from build123d import *

# Parameters (mm, degrees)
F0_W            = 19.812
F0_H            = 19.812
F1_DEPTH        = 31.9532
F2_R            = 3.556
F3_DEPTH        = 25.9334
F4_T1_DEPTH     = 0.8065583261
F4_T3_DEPTH     = 0.8065583261
F4_T5_DEPTH     = 0.8065583261
F4_T7_DEPTH     = 0.8065583261
F4_T9_DEPTH     = 0.8065583261
F4_T11_DEPTH    = 0.8065583261
F4_T13_DEPTH    = 0.8065583261
F4_T15_DEPTH    = 0.8065583261
F4_T17_DEPTH    = 35.2192373947
F4_T19_DEPTH    = 23.0780373947
F4_T21_DEPTH    = 23.0780373947
F5_W            = 0.254
F5_H            = 11.8872
F5_H_2          = 0.254
F5_W_2          = 9.779
F5_H_3          = 19.812
F6_DEPTH        = 1.016
F6_COPIES_COUNT = 4
F7_W            = 0.254
F7_H            = 8.763
F7_H_2          = 0.254
F7_W_2          = 8.763
F8_DEPTH        = 1.016


# Not quite as in the source:
# - a fillet or chamfer that OpenCascade refuses, or shapes differently, is made with other operations: its cross-section is extruded or revolved along the edge and cut away or added
# - a pattern or mirror of a feature is missing from the dataset's text; its kind, count and spacing are read off the source's solid


with BuildPart() as f1:
    # F0 (on Top) → F1 (new body)
    with BuildSketch(Plane.XY):
        Rectangle(F0_W, F0_H)
    extrude(amount=F1_DEPTH)

    # F2 (on face) → F3 (cut)
    with BuildSketch(Plane.XY.offset(31.9532)):
        Circle(F2_R)
    extrude(amount=-F3_DEPTH, mode=Mode.SUBTRACT)

    # F4: chamfer of 0.635 on 12 edges, made by hand

    # F4_s2 → F4_t1 (cut)
    with BuildSketch(Plane(origin=(-6.1806666667, 6.1806666667, -6.1806666667), x_dir=(-0.7071067812, -0.7071067812, 0), z_dir=(-0.5773502692, 0.5773502692, -0.5773502692))):
        Polygon((-0.4490128061, 8.3474527951), (0, 7.5697398018), (0.4490128061, 8.3474527951), align=None)
    extrude(amount=F4_T1_DEPTH, mode=Mode.SUBTRACT)

    # F4_s4 → F4_t3 (cut)
    with BuildSketch(Plane(origin=(-16.8317333333, 16.8317333333, 16.8317333333), x_dir=(-0.7071067812, -0.7071067812, 0), z_dir=(-0.5773502692, 0.5773502692, 0.5773502692))):
        Polygon((-0.4490128061, 17.7422257546), (0, 18.5199387479), (0.4490128061, 17.7422257546), align=None)
    extrude(amount=F4_T3_DEPTH, mode=Mode.SUBTRACT)

    # F4_s6 → F4_t5 (cut)
    with BuildSketch(Plane(origin=(-6.1806666667, -6.1806666667, -6.1806666667), x_dir=(0.7071067812, -0.7071067812, 0), z_dir=(-0.5773502692, -0.5773502692, -0.5773502692))):
        Polygon((0.4490128061, 8.3474527951), (0, 7.5697398018), (-0.4490128061, 8.3474527951), align=None)
    extrude(amount=F4_T5_DEPTH, mode=Mode.SUBTRACT)

    # F4_s8 → F4_t7 (cut)
    with BuildSketch(Plane(origin=(-16.8317333333, -16.8317333333, 16.8317333333), x_dir=(0.7071067812, -0.7071067812, 0), z_dir=(-0.5773502692, -0.5773502692, 0.5773502692))):
        Polygon((0.4490128061, 17.7422257546), (0, 18.5199387479), (-0.4490128061, 17.7422257546), align=None)
    extrude(amount=F4_T7_DEPTH, mode=Mode.SUBTRACT)

    # F4_s10 → F4_t9 (cut)
    with BuildSketch(Plane(origin=(6.1806666667, -6.1806666667, -6.1806666667), x_dir=(0.7071067812, 0.7071067812, 0), z_dir=(0.5773502692, -0.5773502692, -0.5773502692))):
        Polygon((0.4490128061, 8.3474527951), (-0.4490128061, 8.3474527951), (0, 7.5697398018), align=None)
    extrude(amount=F4_T9_DEPTH, mode=Mode.SUBTRACT)

    # F4_s12 → F4_t11 (cut)
    with BuildSketch(Plane(origin=(16.8317333333, -16.8317333333, 16.8317333333), x_dir=(0.7071067812, 0.7071067812, 0), z_dir=(0.5773502692, -0.5773502692, 0.5773502692))):
        Polygon((0.4490128061, 17.7422257546), (-0.4490128061, 17.7422257546), (0, 18.5199387479), align=None)
    extrude(amount=F4_T11_DEPTH, mode=Mode.SUBTRACT)

    # F4_s14 → F4_t13 (cut)
    with BuildSketch(Plane(origin=(6.1806666667, 6.1806666667, -6.1806666667), x_dir=(-0.7071067812, 0.7071067812, 0), z_dir=(0.5773502692, 0.5773502692, -0.5773502692))):
        Polygon((-0.4490128061, 8.3474527951), (0.4490128061, 8.3474527951), (0, 7.5697398018), align=None)
    extrude(amount=F4_T13_DEPTH, mode=Mode.SUBTRACT)

    # F4_s16 → F4_t15 (cut)
    with BuildSketch(Plane(origin=(16.8317333333, 16.8317333333, 16.8317333333), x_dir=(-0.7071067812, 0.7071067812, 0), z_dir=(0.5773502692, 0.5773502692, 0.5773502692))):
        Polygon((-0.4490128061, 17.7422257546), (0.4490128061, 17.7422257546), (0, 18.5199387479), align=None)
    extrude(amount=F4_T15_DEPTH, mode=Mode.SUBTRACT)

    # F4_s18 → F4_t17 (cut)
    with BuildSketch(Plane.XY.offset(-1.6330186974)):
        Polygon((-9.271, 9.906), (-9.906, 9.271), (-9.906, 9.906), align=None)
        Polygon((-9.271, -9.906), (-9.906, -9.271), (-9.906, -9.906), align=None)
        Polygon((9.906, -9.271), (9.271, -9.906), (9.906, -9.906), align=None)
        Polygon((9.906, 9.271), (9.271, 9.906), (9.906, 9.906), align=None)
    extrude(amount=F4_T17_DEPTH, mode=Mode.SUBTRACT)

    # F4_s20 → F4_t19 (cut)
    with BuildSketch(Plane.XZ.offset(-11.5390186974)):
        Polygon((9.906, 31.3182), (9.271, 31.9532), (9.906, 31.9532), align=None)
        Polygon((-9.271, 31.9532), (-9.906, 31.3182), (-9.906, 31.9532), align=None)
        Polygon((9.906, 0.635), (9.271, 0), (9.906, 0), align=None)
        Polygon((-9.271, 0), (-9.906, 0.635), (-9.906, 0), align=None)
    extrude(amount=F4_T19_DEPTH, mode=Mode.SUBTRACT)

    # F4_s22 → F4_t21 (cut)
    with BuildSketch(Plane.YZ.offset(-11.5390186974)):
        Polygon((-9.906, 31.3182), (-9.271, 31.9532), (-9.906, 31.9532), align=None)
        Polygon((9.906, 31.3182), (9.271, 31.9532), (9.906, 31.9532), align=None)
        Polygon((9.906, 0.635), (9.271, 0), (9.906, 0), align=None)
        Polygon((-9.906, 0.635), (-9.271, 0), (-9.906, 0), align=None)
    extrude(amount=F4_T21_DEPTH, mode=Mode.SUBTRACT)

    # F5 (on face) → F6 (cut)
    with BuildSketch(Plane.XZ.offset(9.906)):
        with Locations((0, 26.0096)):
            Rectangle(F5_W, F5_H)
        with Locations((0, 19.939)):
            Rectangle(F5_W, F5_H_2)
        with Locations((-5.0165, 19.939)):
            Rectangle(F5_W_2, F5_H_2)
        with Locations((5.0165, 19.939)):
            Rectangle(F5_W_2, F5_H_2)
        with Locations((0, 9.906)):
            Rectangle(F5_W, F5_H_3)
    f6 = extrude(amount=-F6_DEPTH, mode=Mode.SUBTRACT)

    # F6_copies: F6 ×4 about axis
    f6_copies_axis = Axis((0, 0, 0), (0, 0, 1))
    for i in range(1, F6_COPIES_COUNT):
        add(f6.rotate(f6_copies_axis, i * 360 / F6_COPIES_COUNT), mode=Mode.SUBTRACT)

    # F7 (on face) → F8 (cut)
    with BuildSketch(Plane(origin=(0, 0, 0), x_dir=(1, 0, 0), z_dir=(0, 0, -1))):
        with Locations((0, 4.5085)):
            Rectangle(F7_W, F7_H)
        Rectangle(F7_W, F7_H_2)
        with Locations((-4.5085, 0)):
            Rectangle(F7_W_2, F7_H_2)
        with Locations((4.5085, 0)):
            Rectangle(F7_W_2, F7_H_2)
        with Locations((0, -4.5085)):
            Rectangle(F7_W, F7_H)
    extrude(amount=-F8_DEPTH, mode=Mode.SUBTRACT)


solid = f1.part
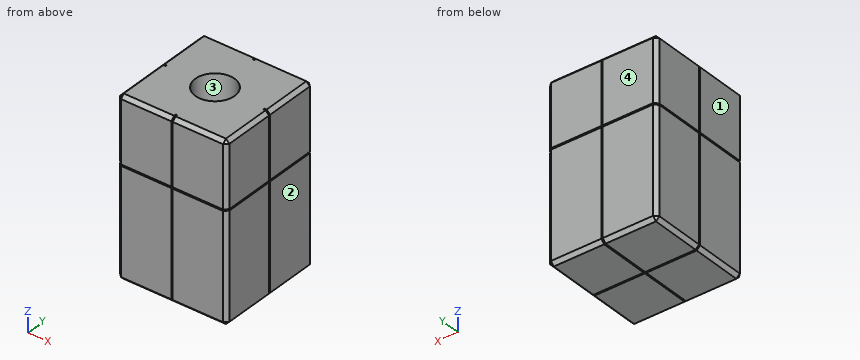
CAD build for the part. Positions are in the model's coordinates, mm. Face numbers are marked on the shaded views. Give positions to 0.01 mm unless a question says otherwise; leave off trailing zeros. Write each loop counter-clockwise with the first axis right and the second up, starting at its lowest first coordinate (ties: lowest second). Pieces come first, ordered by that corner, then holes. Notation, with made-up numbers: (53.25, 53.25) -> (108.25, 53.25) arc R23 ccw to (108.25, 72.25) -> close; hole circle Ø9 at (45, 29.5). An arc over 180 degrees is marked (long way). Return JSON: item names as keys, results as strings.
Item 1: Band-saw the part on A-A (z = 9). List the corners of the cut face in (x, y), then the cut area to 3 significant figures.
Answer below:
{"outline": "(-9.91, -9.27) -> (-9.27, -9.91) -> (-0.13, -9.91) -> (-0.13, -8.89) -> (0.13, -8.89) -> (0.13, -9.91) -> (9.27, -9.91) -> (9.91, -9.27) -> (9.91, -0.13) -> (8.89, -0.13) -> (8.89, 0.13) -> (9.91, 0.13) -> (9.91, 9.27) -> (9.27, 9.91) -> (0.13, 9.91) -> (0.13, 8.89) -> (-0.13, 8.89) -> (-0.13, 9.91) -> (-9.27, 9.91) -> (-9.91, 9.27) -> (-9.91, 0.13) -> (-8.89, 0.13) -> (-8.89, -0.13) -> (-9.91, -0.13) -> close; hole circle Ø7.11 at (0, 0)", "area": "351 mm2"}
Item 2: Band-saw the part on C-C (x = 1.75). List the corners of the cut face in (y, z) (3 decimals).
Answer below:
{"outline": "(-9.906, 0.635) -> (-9.271, 0) -> (-0.127, 0) -> (-0.127, 1.016) -> (0.127, 1.016) -> (0.127, 0) -> (9.271, 0) -> (9.906, 0.635) -> (9.906, 19.812) -> (8.89, 19.812) -> (8.89, 20.066) -> (9.906, 20.066) -> (9.906, 31.318) -> (9.271, 31.953) -> (3.096, 31.953) -> (3.096, 6.02) -> (-3.096, 6.02) -> (-3.096, 31.953) -> (-9.271, 31.953) -> (-9.906, 31.318) -> (-9.906, 20.066) -> (-8.89, 20.066) -> (-8.89, 19.812) -> (-9.906, 19.812) -> close"}
Item 3: Drill centre lines: probe 1 along Z at (x, y) = (9, 4.5); probe 2 along Y at (x, z) = (0, 14.25); probe 3 along Y at (x, z) = (9, 27). Where is each one in solid material? Low to high.
Answer below:
{"probe 1": "z = 0 to 19.81, 20.07 to 31.95", "probe 2": "y = -8.89 to -3.56, 3.56 to 8.89", "probe 3": "y = -9.91 to -0.13, 0.13 to 9.91"}
Item 4: Band-saw the part on B-B (y = -3). List the corners of the cut face in (x, z) (3 decimals).
Answer below:
{"outline": "(-9.906, 0.635) -> (-9.271, 0) -> (-0.127, 0) -> (-0.127, 1.016) -> (0.127, 1.016) -> (0.127, 0) -> (9.271, 0) -> (9.906, 0.635) -> (9.906, 19.812) -> (8.89, 19.812) -> (8.89, 20.066) -> (9.906, 20.066) -> (9.906, 31.318) -> (9.271, 31.953) -> (1.909, 31.953) -> (1.909, 6.02) -> (-1.909, 6.02) -> (-1.909, 31.953) -> (-9.271, 31.953) -> (-9.906, 31.318) -> (-9.906, 20.066) -> (-8.89, 20.066) -> (-8.89, 19.812) -> (-9.906, 19.812) -> close"}
Item 5: Two-plate mould, pull along X, no slides. Class the marked faces 1, 2, 3 and 4: +X half, -X half, draft (parallel to the pull), parting line (faces both ways), or undercut.
Answer below:
{"face 1": "-X half", "face 2": "+X half", "face 3": "undercut", "face 4": "draft"}
